Design review of the part built by this model. Coordinates are the model's own, in mm. Face numbers are marked on the shaded views. A direction names the side the tool comes from. Give positions to 0.01 mm unless a question says otherwise; leave off trailing zeros. Write each loop counter-clockwise with the first axis right and the second up, starting at its lowest first coordinate (ties: lowest second). Pieces come first, ordered by that corner, then holes. Notation, with made-up numbers: (-27.5, 23) -> (24.5, 23) arc R36 cw to (24.5, 60) -> close; hole circle Ø4 at (57.5, 29.5). An arc over 180 degrees is marked (long way). Write each question's results on one line, items separated by ' | '. Start each with the question number.
(1) For the marked faces 1, 2, 3, 4 and 5, list the 3-axis set-ups (+Z, -Z, +X, -X, +Y, -Y) from which the entire face can be reached by the end or side of a thin tool; tool diameter is ignored.
(2) Clearance check with flat-ended pins moving along their axes: pin 1 (1.8 mm diameter, centred on x = 0, y = 2, fed in from -Z); pin 2 (22 mm diameter, centred on x = -9, z = -5, fed in from +Y) (3 decimals); pin 3 (3 mm diameter, centred on y = 7.5, z = 14.5, fed in from +X); pin 4 (2 mm diameter, centred on x = 1, y = 5.5, fed in from +Z). State where each tip first meets the part, or that it passes through.
(3) Take a section at C-C (y = 4.25). State the section outline as (x, z) points (3 decimals), plus the area to 3 significant figures.
(4) To check wall thickness, follow probe 1 along Z at (x, y) = (0, 9.3) (3 decimals); probe 2 along Z at (x, y) = (-13, 8.5); probe 3 along Z at (x, y) = (0, 7.35) (3 decimals). State the ranges of each line that lie inside material, in increasing order.
(5) Mouldability with a two-part tool opening along Z and no side actions: class the marked faces 6, 7 and 8 as released by +Z, released by -Z, zero draft, split by the parting line, or undercut.
from build123d import *

# Parameters (mm, degrees)
BOSS_EXTRUDE1_DEPTH = 10.795
SKETCH2_R           = 22.8346
BOSS_EXTRUDE2_DEPTH = 7.2898
SKETCH3_R           = 22.0726
SKETCH3_R_2         = 16.51
CUT_EXTRUDE1_DEPTH  = 5.08
SKETCH4_R           = 12.065
CUT_EXTRUDE2_DEPTH  = 11.795
SKETCH5_R           = 18.1356
SKETCH5_R_2         = 14.8844
CUT_EXTRUDE5_DEPTH  = 2.54
FILLET1_R           = 1.27
FILLET2_R           = 1.27
FILLET3_R           = 1.27


with BuildPart() as part:
    # Sketch1 → Boss-Extrude1 (new body)
    with BuildSketch(Plane(origin=(0, 0, 0), x_dir=(1, 0, 0), z_dir=(0, 1, 0))):
        Polygon((-7.339781299, 15.8115), (7.339781299, 15.8115), (15.8115, 6.35), (15.8115, -6.35), (7.339781299, -15.8115), (-7.339781299, -15.8115), (-15.8115, -6.35), (-15.8115, 6.35), align=None)
    extrude(amount=BOSS_EXTRUDE1_DEPTH)

    # Sketch2 → Boss-Extrude2 (add)
    with BuildSketch(Plane(origin=(0, 3.5052, 0), x_dir=(-1, 0, 0), z_dir=(0, -1, 0))):
        Circle(SKETCH2_R)
    extrude(amount=-BOSS_EXTRUDE2_DEPTH)

    # Sketch3 → Cut-Extrude1 (cut)
    with BuildSketch(Plane(origin=(0, 10.795, 0), x_dir=(1, 0, 0), z_dir=(0, 1, 0))):
        Circle(SKETCH3_R)
        Circle(SKETCH3_R_2, mode=Mode.SUBTRACT)
    extrude(amount=-CUT_EXTRUDE1_DEPTH, mode=Mode.SUBTRACT)

    # Sketch4 → Cut-Extrude2 (cut, through all)
    with BuildSketch(Plane.XZ):
        Circle(SKETCH4_R)
    extrude(amount=-CUT_EXTRUDE2_DEPTH, mode=Mode.SUBTRACT)

    # Sketch5 → Cut-Extrude5 (cut)
    with BuildSketch(Plane(origin=(0, 10.795, 0), x_dir=(1, 0, 0), z_dir=(0, 1, 0))):
        Circle(SKETCH5_R)
        Circle(SKETCH5_R_2, mode=Mode.SUBTRACT)
    extrude(amount=-CUT_EXTRUDE5_DEPTH, mode=Mode.SUBTRACT)

    # Fillet1
    fillet1_edges = [part.edges().sort_by_distance(p)[0] for p in [
        (-14.8844, 10.795, 0),
    ]]
    fillet(fillet1_edges, radius=FILLET1_R)

    # Fillet2
    fillet2_edges = [part.edges().sort_by_distance(p)[0] for p in [
        (-16.51, 8.255, 0),
    ]]
    fillet(fillet2_edges, radius=FILLET2_R)

    # Fillet3
    fillet3_edges = [part.edges().sort_by_distance(p)[0] for p in [
        (22.8346, 3.5052, 0),
    ]]
    fillet(fillet3_edges, radius=FILLET3_R)


solid = part.part
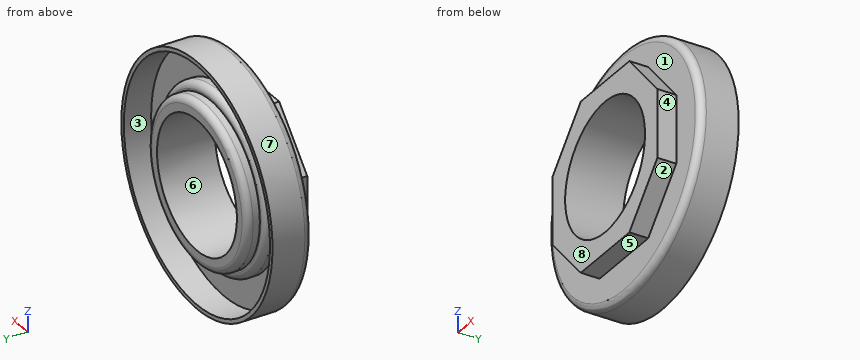
Report:
1) face 1: -Y | face 2: -Z, +X, -Y | face 3: +Y | face 4: +Z, -Z, +X, -Y | face 5: -Z, +X, -X, -Y
2) pin 1: z = -15.81 | pin 2: y = 10.795 | pin 3: x = 18.77 | pin 4: z = 22.83
3) outline: circle Ø45.442 at (0, 0); hole circle Ø24.13 at (0, 0) | area: 1,160 mm2
4) probe 1: -22.835 to -22.073, -14.884 to -12.065, 12.065 to 14.884, 22.073 to 22.835 | probe 2: -18.77 to -17.84, -7.25 to 7.25, 17.84 to 18.77 | probe 3: -22.835 to -22.073, -16.456 to -12.065, 12.065 to 16.456, 22.073 to 22.835
5) face 6: undercut | face 7: split by the parting line | face 8: zero draft
